Part model, mm, in its own coordinate system. Face numbers are marked on the shaded views. A direction names the side the tool comes from. Round coordinates to 2 decimals unless told otherwise and drop trailing zeros. Loops run counter-clockwise (first coordinate to the right, second up) from the corner with the lowest first, then second, coordinate; pieces in that order, holes last. Notation, with made-up numbers: (-9, -1) - (7, -1) arc R5 cw to (7, 6) - close; hole circle Ø3 at (77, 9.25). An arc over 180 degrees is marked (long way). Write each question's results on one line, items separated by ' | '. Start each with the question number.
(1) Tool access for the marked faces 1 and 2: list every direction of +Z, -Z, +X, -X, +Y, -Y with a clear straight run to the whole face (end or side of a thin tool).
(2) Cut at C-C, the plane z = 10.25. List the corners of the cut face in (x, y).
(3) Mould opens along Z. For the marked faces 3, 4 and 5 say: released by +Z, released by -Z, zero draft, split by the parting line, or undercut.
(4) Cut at B-B, the plane x = 8. List the corners of the cut face in (y, z).
(5) Cut at D-D, the plane x = 13. List the corners of the cut face in (y, z).
(6) Drill centre lines: L1, parallel to Y at x = 10.25, z = 12.75; L2, parallel to Z at x = 8.25, y = 66.65; L3, parallel to X at y = 66.05, z = 12.25. Where is each one in solid material? Low to high.
(7) Cut at A-A, the plane y = 65.7. List the corners of the cut face in (x, z).
(8) Flat gauge pin, fed straight in: P1, Ø2, axis at x = 9.5, z = 11.5, coming from the +Y side. Where does the tip first touch, or does it go through?
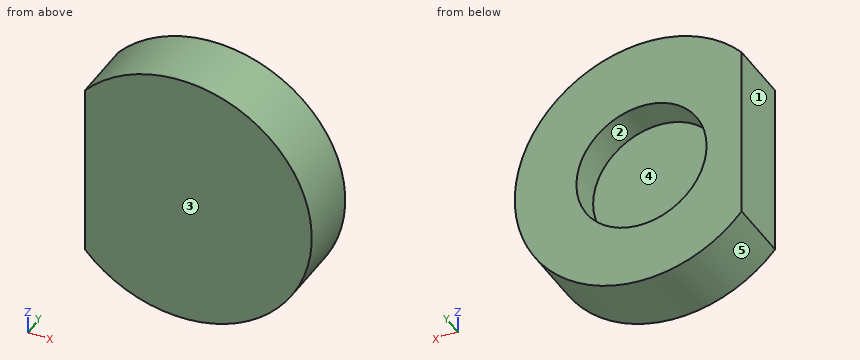
from build123d import *

# Parameters (mm, degrees)
CIRCLE008_AS_DRAWN_R                      = 2
EXTRUDE015_DEPTH                          = 2
EXTRUDE015_ONTO_CIRCLE008_ROLL_ANGLE      = 90
EXTRUDE015_ONTO_CIRCLE008_PLACEMENT_ANGLE = 180
RECTANGLE005_AS_DRAWN_W                   = 5.41291
RECTANGLE005_AS_DRAWN_H                   = 8.044928
EXTRUDE010_DEPTH                          = 3
EXTRUDE010_ONTO_RECTANGLE005_ROLL_ANGLE   = 90
CIRCLE002_AS_DRAWN_R                      = 4
EXTRUDE009_DEPTH                          = 2
EXTRUDE009_ONTO_CIRCLE002_ROLL_ANGLE      = 90


with BuildPart() as extrude015:
    # Circle008 as drawn → Extrude015 (new)
    with BuildSketch(Plane.XY):
        Circle(CIRCLE008_AS_DRAWN_R)
    extrude(amount=EXTRUDE015_DEPTH)


with BuildPart() as extrude015_1:
    # Extrude015 onto Circle008 roll: moved
    add(extrude015.part.rotate(Axis((0, 0, 0), (1, 0, 0)), EXTRUDE015_ONTO_CIRCLE008_ROLL_ANGLE))


with BuildPart() as extrude015_2:
    # Extrude015 onto Circle008 placement: moved
    add(extrude015_1.part.moved(Location((9.579189, 64.900139, 11.27318))).rotate(Axis((9.579189, 64.900139, 11.27318), (0, 0, 1)), EXTRUDE015_ONTO_CIRCLE008_PLACEMENT_ANGLE))


with BuildPart() as extrude015_3:
    # Extrude015 placement: moved
    add(extrude015_2.part.moved(Location((0, 1, 0))))


with BuildPart() as extrude010:
    # Rectangle005 as drawn → Extrude010 (new)
    with BuildSketch(Plane.XY):
        with Locations((-2.706455, -4.022464)):
            Rectangle(RECTANGLE005_AS_DRAWN_W, RECTANGLE005_AS_DRAWN_H)
    extrude(amount=-EXTRUDE010_DEPTH)


with BuildPart() as extrude010_1:
    # Extrude010 onto Rectangle005 roll: moved
    add(extrude010.part.rotate(Axis((0, 0, 0), (1, 0, 0)), EXTRUDE010_ONTO_RECTANGLE005_ROLL_ANGLE))


with BuildPart() as extrude010_2:
    # Extrude010 onto Rectangle005 placement: moved
    add(extrude010_1.part.moved(Location((56.902615, 1.09014, 40.499655))))


with BuildPart() as extrude010_3:
    # Extrude010 placement: moved
    add(extrude010_2.part.moved(Location((0, -0.5, 0))))


with BuildPart() as obj1:
    # Circle002 as drawn → Extrude009 (new)
    with BuildSketch(Plane.XY):
        Circle(CIRCLE002_AS_DRAWN_R)
    extrude(amount=-EXTRUDE009_DEPTH)


with BuildPart() as obj1_1:
    # Extrude009 onto Circle002 roll: moved
    add(obj1.part.rotate(Axis((0, 0, 0), (1, 0, 0)), EXTRUDE009_ONTO_CIRCLE002_ROLL_ANGLE))


with BuildPart() as obj1_2:
    # Extrude009 onto Circle002 placement: moved
    add(obj1_1.part.moved(Location((59.872219, 1.090141, 36.55234))))

    # Cut: cut Extrude010
    add(extrude010_3.part, mode=Mode.SUBTRACT)


with BuildPart() as obj1_3:
    # Cut placement: moved
    add(obj1_2.part.moved(Location((-50.399612, 63.810001, -25.16555))))

    # Cut002: cut Extrude015
    add(extrude015_3.part, mode=Mode.SUBTRACT)


solid = obj1_3.part
A:
1) face 1: +Z, -Z, -X, +Y, -Y | face 2: +Y
2) outline: (6.5, 64.9) - (13.31, 64.9) - (13.31, 66.9) - (11.3, 66.9) - (11.3, 65.9) - (7.86, 65.9) - (7.86, 66.9) - (6.5, 66.9) - close
3) face 3: zero draft | face 4: undercut | face 5: split by the parting line
4) outline: (64.9, 7.67) - (66.9, 7.67) - (66.9, 10.05) - (65.9, 10.05) - (65.9, 12.5) - (66.9, 12.5) - (66.9, 15.11) - (64.9, 15.11) - close
5) outline: (64.9, 9.5) - (66.9, 9.5) - (66.9, 13.27) - (64.9, 13.27) - close
6) L1: 64.9 to 65.9 | L2: 7.58 to 9.78, 12.77 to 15.2 | L3: 6.5 to 7.83, 11.32 to 13.38
7) outline: (6.5, 8.71) arc R4 ccw (long way) to (6.5, 14.07) - close
8) P1: y = 65.9
